The listing builds one solid part. Answer for the finished solid, in the listing's coordinates (mm). A direction names the side the tool comes from. Round coordinates to 2 decimals unless told otherwise and drop trailing zeros. Loops run counter-clockwise (first coordinate to the right, second up) from the corner with the lowest first, then second, coordinate; pieces in that order, holes last. Notation, with made-up numbers: (-12.75, 35) -> (38.25, 35) arc R24 cw to (38.25, 70) -> close; hole circle Ø4 at (72, 72). An arc over 180 degrees is marked (long way). Answer in a Markdown table with one row per item. Add a question column.
```python
from build123d import *

# Parameters (mm, degrees)
F1_DEPTH = 40
F2_R     = 13
F3_T     = -2.5
F4_SIZE  = 2


with BuildPart() as f1:
    # F0 (on Top) → F1 (new body)
    with BuildSketch(Plane.XY):
        Polygon((-13.856406, 63), (-13.856406, 8), (-61.487804, -19.5), (-47.631397, -43.5), (0, -16), (47.631397, -43.5), (61.487804, -19.5), (13.856406, 8), (13.856406, 63), align=None)
    extrude(amount=F1_DEPTH)

    # F2
    f2_edges = [f1.edges().sort_by_distance(p)[0] for p in [
        (-47.631397, -43.5, 20),
        (-61.487804, -19.5, 20),
        (0, -16, 20),
        (47.631397, -43.5, 20),
        (61.487804, -19.5, 20),
        (13.856406, 8, 20),
        (13.856406, 63, 20),
        (-13.856406, 63, 20),
        (-13.856406, 8, 20),
    ]]
    fillet(f2_edges, radius=F2_R)

    # F3
    f3_openings = [f1.faces().sort_by_distance(p)[0] for p in [
        (0, 0, 40),
    ]]
    offset(amount=F3_T, openings=f3_openings)

    # F4
    f4_edges = [f1.edges().sort_by_distance(p)[0] for p in [
        (-21.436533, -28.376388, 0),
        (-46.237715, -38.298705, 0),
        (0, -18.011107, 0),
        (-54.5596, -31.5, 0),
        (21.436533, -28.376388, 0),
        (-56.286509, -20.893683, 0),
        (46.237715, -38.298705, 0),
        (-35.29294, -4.376388, 0),
        (54.5596, -31.5, 0),
        (-15.598076, 9.005553, 0),
        (56.286509, -20.893683, 0),
        (-13.856406, 32.752777, 0),
        (35.29294, -4.376388, 0),
        (-10.048795, 59.192388, 0),
        (15.598076, 9.005553, 0),
        (0, 63, 0),
        (13.856406, 32.752777, 0),
        (10.048795, 59.192388, 0),
    ]]
    chamfer(f4_edges, length=F4_SIZE)


solid = f1.part
```
Item 1: The mould has two halves that part along X. Classify faces 4 (the cylindrical face through (53.9, -21.65, 21.51)), 5 (the conical face through (-14.89, 8.71, 1.24)), 6 (the conical face through (54.722, -21.442, 0.347)): +X half, -X half, draft (parallel to the pull), parting line (faces both ways), or undercut.
Item 2: Flat-ended cylindrical pins translate along their axes: P1, Ø2, axis at y = 31, z = 19.5, coming from the +X side; P2, Ø3, axis at y = 4.5, z = 11.5, coming from the -X side; P3, Ø5, axis at y = -21, z = 36, coming from the +X side. Find the tip coordinate at first contact, or state that the pin passes through.
Item 3: For faces 1 (the flat face through (21.72, -27.4, 1.01)), 2 (the flat face through (-22.896, -26.332, 20.988)), 3 (the flat face through (-34.591, -5.11, 1.014)), determine the directions among +Z, -Z, +X, -X, +Y, -Y from which every point of the face is accessible in a straight line to the end or side of a thin tool.
Item 4: Section B-B, the plane x = 25.5 is taken. Write down the section's boundary in (y, z).
Item 5: Consider L1, parallel to X at y = 39.5, z = 15.5; L2, parallel to X at y = -21, z = 37; L3, parallel to Y at x = -26.5, z = 4. Determine where each line is inside the solid, lowest interval first. Write a range as from..to.
Item 6: Section A-A, the plane y = 33 is taken. Write down the section's boundary in (x, z).
Here are the results:
| question | item | result |
|---|---|---|
| 1 | face 4 | undercut |
| 1 | face 5 | -X half |
| 1 | face 6 | +X half |
| 2 | P1 | stops at x = 13.86 |
| 2 | P2 | stops at x = -22.52 |
| 2 | P3 | stops at x = 56.71 |
| 3 | face 1 | -Z, -Y |
| 3 | face 2 | +Z |
| 3 | face 3 | -Z, -X, +Y |
| 4 | outline | (-30.72, 2) -> (-28.41, 0) -> (-1.03, 0) -> (1.28, 2) -> (1.28, 40) -> (-1.61, 40) -> (-1.61, 2.5) -> (-27.84, 2.5) -> (-27.84, 40) -> (-30.72, 40) -> close |
| 5 | L1 | x = -13.86..-11.36, 11.36..13.86 |
| 5 | L2 | x = -56.31..-53.71, -13.66..-8.66, 8.66..13.66, 53.71..56.31 |
| 5 | L3 | y = -31.3..-28.41, -2.19..0.7 |
| 6 | outline | (-13.86, 2) -> (-11.86, 0) -> (11.86, 0) -> (13.86, 2) -> (13.86, 40) -> (11.36, 40) -> (11.36, 2.5) -> (-11.36, 2.5) -> (-11.36, 40) -> (-13.86, 40) -> close |
